from build123d import *

# Parameters (mm, degrees)
EXTRUDE_1_DEPTH     = 22.5
SKETCH_2_R          = 1
CUT_EXTRUDE_1_DEPTH = 4
CHAMFER_1_SIZE      = 0.5


with BuildPart() as part:
    # 草图1 → 凸台-拉伸1 (new body)
    with BuildSketch(Plane(origin=(0, 0, 0), x_dir=(1, 0, 0), z_dir=(0, 1, 0))):
        Polygon((-8.5, 3.25), (-8.5, -3.25), (-3.5, -3.25), (-3.5, -2.25), (-2.5, -2.25), (-2.5, -1.25), (-3.5, -1.25), (-3.5, -0.25), (3.5, -0.25), (3.5, -1.25), (2.5, -1.25), (2.5, -2.25), (3.5, -2.25), (3.5, -3.25), (8.5, -3.25), (8.5, 3.25), align=None)
    extrude(amount=EXTRUDE_1_DEPTH)

    # 草图2 → 切除-拉伸1 (cut)
    with BuildSketch(Plane(origin=(0, 0, -3.25), x_dir=(-1, 0, 0), z_dir=(0, 0, -1))):
        with Locations((6, 15.25)):
            Circle(SKETCH_2_R)
        with Locations(Location((6, 7.25, 0), (0, 0, 180))):
            Circle(SKETCH_2_R)
        with Locations((-6, 7.25)):
            Circle(SKETCH_2_R)
        with Locations(Location((-6, 15.25, 0), (0, 0, 180))):
            Circle(SKETCH_2_R)
    extrude(amount=-CUT_EXTRUDE_1_DEPTH, mode=Mode.SUBTRACT)

    # 倒角1
    chamfer_1_edges = [part.edges().sort_by_distance(p)[0] for p in [
        (-8.5, 11.25, -3.25),
        (8.5, 11.25, -3.25),
    ]]
    chamfer(chamfer_1_edges, length=CHAMFER_1_SIZE)


solid = part.part
Build history of the part. All positions in model axes, mm. A direction names the side the tool comes from. Give positions to 0.01 mm unless a question says otherwise; leave off trailing zeros. Order: outer loops, then holes, each group sorted by start corner. A loop starts at its lowest first (then second) coordinate and runs counter-clockwise, first axis right, second up. Notation, with made-up numbers: M 89.25,-22 L 118.25,-22 A16 cw 118.25,-7 Z; hole C 33,-39 d4. An arc over 180 degrees is marked long. Put each result on its own line as item: value.
Item 1: Slice it at C-C, the plane x = 6. Write the cut outline in (y, z), plus the area to 3 significant figures.
From the geometry:
outline: M 0,-3.25 L 6.25,-3.25 L 6.25,0.75 L 8.25,0.75 L 8.25,-3.25 L 14.25,-3.25 L 14.25,0.75 L 16.25,0.75 L 16.25,-3.25 L 22.5,-3.25 L 22.5,3.25 L 0,3.25 Z
area: 130 mm2
Item 2: Slice it at A-A, the plane z = 1. Write the cut outline in (x, y), plus the area to 3 significant figures.
From the geometry:
outline: M -8.5,0 L -3.5,0 L -3.5,22.5 L -8.5,22.5 Z; M 3.5,0 L 8.5,0 L 8.5,22.5 L 3.5,22.5 Z
area: 225 mm2
Item 3: Slice it at B-B, the plane y = 5.75. Write the cut outline in (x, z).
From the geometry:
outline: M -8.5,-2.75 L -8,-3.25 L 8,-3.25 L 8.5,-2.75 L 8.5,3.25 L 3.5,3.25 L 3.5,2.25 L 2.5,2.25 L 2.5,1.25 L 3.5,1.25 L 3.5,0.25 L -3.5,0.25 L -3.5,1.25 L -2.5,1.25 L -2.5,2.25 L -3.5,2.25 L -3.5,3.25 L -8.5,3.25 Z
Item 4: Two-plate mould, pull along Z, no slides. Class faces 5 (the flat face through (3, 11, 2.25)), 6 (the flat face through (-3.5, 11, 1)), 7 (the flat face through (0, 22.5, 0)): +Z half, -Z half, draft (parallel to the pull), parting line (faces both ways), or undercut.
From the geometry:
face 5: +Z half
face 6: undercut
face 7: draft
Item 5: 3-axis set-ups, long thin cutter, end or side, ignore diameter. For faces 1 (the flat face through (3.5, 11, 3)), 2 (the flat face through (-3, 11, 1.25)), 3 (the cylindrical face through (6.13, 8.24, -1.28)), 4 (the flat face through (-6, 11, 3.25)): which of +Z, -Z, +X, -X, +Y, -Y reach the whole face in a straight line?
From the geometry:
face 1: +Z, +Y, -Y
face 2: +Y, -Y
face 3: -Z
face 4: +Z, +X, -X, +Y, -Y
Item 6: Slice it at D-D, the plane y = 15.25. Write the cut outline in (x, z), plus the area to 4 significant figures.
From the geometry:
outline: M -8.5,-2.75 L -8,-3.25 L -7,-3.25 L -7,0.75 L -5,0.75 L -5,-3.25 L 5,-3.25 L 5,0.75 L 7,0.75 L 7,-3.25 L 8,-3.25 L 8.5,-2.75 L 8.5,3.25 L 3.5,3.25 L 3.5,2.25 L 2.5,2.25 L 2.5,1.25 L 3.5,1.25 L 3.5,0.25 L -3.5,0.25 L -3.5,1.25 L -2.5,1.25 L -2.5,2.25 L -3.5,2.25 L -3.5,3.25 L -8.5,3.25 Z
area: 75.25 mm2
Item 7: Probe line 1 (Y direction, x = -6, z = -0.55); line 2 (X direction, y = 7, z = 1.75); line 3 (X direction, y = 7.75, z = -2.25). List the from-to ranges inside material, lowest first. Write a range as [from, to].
From the geometry:
line 1: y = [0, 6.25], [8.25, 14.25], [16.25, 22.5]
line 2: x = [-8.5, -2.5], [2.5, 8.5]
line 3: x = [-8.5, -6.87], [-5.13, 5.13], [6.87, 8.5]
Item 8: Flat gauge pins, fed straight in: pin 1 Ø3.5 at (x, y) = (0, 11.5) entering from +Z; pin 2 Ø0.8 at (x, y) = (-3, 7) entering from +Z. Where does each tip first touch, or does it go through?
From the geometry:
pin 1: stops at z = 0.25
pin 2: stops at z = 2.25
